```python
from build123d import *

# Parameters (mm, degrees)
F1_DEPTH = 25
F2_DEPTH = 7
F3_DEPTH = 15


with BuildPart() as f1:
    # F0 (on Front) → F1 (new body)
    with BuildSketch(Plane.XZ):
        with BuildLine():
            Line((0, 27.5), (0, 40))
            ThreePointArc((0, 40), (-40, 0), (0, -40))
            Line((0, -40), (0, -27.5))
            ThreePointArc((0, -27.5), (-27.5, 0), (0, 27.5))
        make_face()
        with BuildLine():
            Line((0, 12.5), (0, 27.5))
            ThreePointArc((0, 27.5), (-27.5, 0), (0, -27.5))
            Line((0, -27.5), (0, -12.5))
            ThreePointArc((0, -12.5), (-12.5, 0), (0, 12.5))
        make_face()
    extrude(amount=F1_DEPTH)

    # F0 (on Front) → F2 (join)
    with BuildSketch(Plane.XZ):
        with BuildLine():
            ThreePointArc((0, -40), (-40, 0), (0, 40))
            Line((0, 40), (0, 50))
            ThreePointArc((0, 50), (-50, 0), (0, -50))
            Line((0, -50), (0, -40))
        make_face()
    extrude(amount=F2_DEPTH)

    # F0 (on Front) → F3 (cut)
    with BuildSketch(Plane.XZ):
        with BuildLine():
            Line((0, 12.5), (0, 27.5))
            ThreePointArc((0, 27.5), (-27.5, 0), (0, -27.5))
            Line((0, -27.5), (0, -12.5))
            ThreePointArc((0, -12.5), (-12.5, 0), (0, 12.5))
        make_face()
    extrude(amount=F3_DEPTH, mode=Mode.SUBTRACT)


solid = f1.part
```
Geometry check sheet. Reference: the model listing, model coordinates, mm. A direction names the side the tool comes from. Round coordinates to 2 decimals unless told otherwise and drop trailing zeros. Order: outer loops, then holes, each group sorted by start corner. A loop starts at its lowest first (then second) coordinate and runs counter-clockwise, first axis right, second up. Notation, with made-up numbers: (58.25, 86.5) -> (98.25, 86.5) arc R16 cw to (98.25, 116.5) -> close; hole circle Ø1 at (65.25, -34). An arc over 180 degrees is marked (long way). Return JSON: item names as keys, results as strings. Group by question number.
Q1. Material ranges on probe 1 along Y at (x, z) = (-20.5, -36.5); probe 2 along Y at (x, z) = (-17, -2.5); probe 3 along Z at (x, y) = (-9, -22), recorded low to high. Write a range as from..to.
Q2. Section check A-A, the plane z = 0. Record the boundary of the cut face in (x, y), plus the area to 4 significant figures.
Q3. Section check B-B, the plane x = -11. Record the boundary of the cut face in (y, z) (3 decimals).
Q4. Tool access check on faces 5 (the cylindrical face through (-27.493, -7.395, 0.605)), 6 (the flat face through (-40, -7, 4)), 7 (the flat face through (-31, 0, 1)). Record the directions out of +Z, -Z, +X, -X, +Y, -Y that give a thin tool (end or side, any length) a straight path to the whole face; none if there is none.
Q5. Section check D-D, the plane x = -38. Record the boundary of the cut face in (y, z).
Q6. Release check for a two-part mould opening along Z. For faces 1 (the cylindrical face through (-12.497, -19.93, -0.275)), 2 (the flat face through (-20, -25, 1)), 3 (the flat face through (-14, -15, 0)), 4 (the cylindrical face through (-49.988, -3.451, 1.099)) record: released by +Z, released by -Z, zero draft, split by the parting line, or undercut.
Q7. Gauge pin test, flat ends, axial feed: pin 1 (3 mm diameter, centred on x = -37.5, y = -20.5, fed in from +Z); pin 2 (6 mm diameter, centred on x = -38.5, y = -9, fed in from -Z); pin 3 (12 mm diameter, centred on y = -8, z = 25, fed in from -X); pin 4 (12 mm diameter, centred on x = -33.5, z = 14.5, fed in from +Y). Record the tip position at first contact, or that the pin passes through.
Q8. Section check C-C, the plane y = -11.25. Record the boundary of the cut face in (x, z), plus the area to 3 significant figures.
Numbers:
{
 "1": {"probe 1": "-7..0", "probe 2": "-25..-15", "probe 3": "-38.97..-8.67, 8.67..38.97"},
 "2": {"outline": "(-50, -7) -> (-40, -7) -> (-40, -25) -> (-12.5, -25) -> (-12.5, -15) -> (-27.5, -15) -> (-27.5, 0) -> (-50, 0) -> close", "area": "532.5 mm^2"},
 "3": {"outline": "(-25, -38.458) -> (-7, -38.458) -> (-7, -48.775) -> (0, -48.775) -> (0, -25.204) -> (-15, -25.204) -> (-15, -5.937) -> (-25, -5.937) -> close; (-25, 5.937) -> (-15, 5.937) -> (-15, 25.204) -> (0, 25.204) -> (0, 48.775) -> (-7, 48.775) -> (-7, 38.458) -> (-25, 38.458) -> close"},
 "4": {"face 5": "+X, +Y", "face 6": "-X, -Y", "face 7": "+Z, -Z, +X, -X, +Y"},
 "5": {"outline": "(-25, -12.49) -> (-7, -12.49) -> (-7, -32.5) -> (0, -32.5) -> (0, 32.5) -> (-7, 32.5) -> (-7, 12.49) -> (-25, 12.49) -> close"},
 "6": {"face 1": "undercut", "face 2": "zero draft", "face 3": "undercut", "face 4": "split by the parting line"},
 "7": {"pin 1": "z = 17.44", "pin 2": "z = -34.42", "pin 3": "x = -46.21", "pin 4": "y = 0"},
 "8": {"outline": "(0, -40) -> (0, -27.5) arc R27.5 cw to (0, 27.5) -> (0, 40) arc R40 ccw to start", "area": "1,330 mm^2"}
}
